from build123d import *

# Parameters (mm, degrees)
BOSS_EXTRUDE1_DEPTH = 0.254
SKETCH2_R           = 4.699
CUT_EXTRUDE1_DEPTH  = 1.254
SKETCH3_W           = 2.54
SKETCH3_H           = 0.635
CUT_EXTRUDE2_DEPTH  = 1.254
SKETCH5_OUTSIDE_W   = 121.447
SKETCH5_OUTSIDE_H   = 109.618
CUT_EXTRUDE5_DEPTH  = 1.254


with BuildPart() as part:
    # Sketch1 → Boss-Extrude1 (new body)
    with BuildSketch(Plane.XY):
        with BuildLine():
            Line((67.21146711, 76.191723231), (8.696654013, 17.676910134))
            Line((8.696654013, 17.676910134), (7.228954972, 14.133571205))
            ThreePointArc((7.228954972, 14.133571205), (14.666587579, 6.075099489), (15.105587123, -4.88230096))
            Line((15.105587123, -4.88230096), (18.648926052, -6.35))
            Line((18.648926052, -6.35), (101.401368334, -6.35))
            ThreePointArc((101.401368334, -6.35), (93.866160503, 38.880636728), (67.21146711, 76.191723231))
        make_face()
        with BuildLine():
            Line((88.672924278, 6.35), (27.86051193, 6.35))
            ThreePointArc((27.86051193, 6.35), (26.399857642, 10.93517908), (24.190484974, 15.210228852))
            Line((24.190484974, 15.210228852), (67.191354125, 58.211098004))
            ThreePointArc((67.191354125, 58.211098004), (82.13289044, 34.020557137), (88.672924278, 6.35))
        make_face(mode=Mode.SUBTRACT)
    extrude(amount=BOSS_EXTRUDE1_DEPTH)

    # Sketch2 → Cut-Extrude1 (cut, through all)
    with BuildSketch(Plane.XY.offset(0.254)):
        with Locations((22.225, 0)):
            Circle(SKETCH2_R)
        with Locations((36.195, 0)):
            Circle(SKETCH2_R)
        with Locations((61.722, 0)):
            Circle(SKETCH2_R)
        with Locations((75.692, 0)):
            Circle(SKETCH2_R)
        with Locations((95.25, 0)):
            Circle(SKETCH2_R)
        with Locations((15.715448212, 15.715448212)):
            Circle(SKETCH2_R)
        with Locations((25.593729945, 25.593729945)):
            Circle(SKETCH2_R)
        with Locations((43.644044748, 43.644044748)):
            Circle(SKETCH2_R)
        with Locations((53.522326482, 53.522326482)):
            Circle(SKETCH2_R)
        with Locations((92.004434954, 24.652514046)):
            Circle(SKETCH2_R)
        with Locations((82.48891971, 47.625)):
            Circle(SKETCH2_R)
        with Locations((67.351920908, 67.351920908)):
            Circle(SKETCH2_R)
    extrude(amount=-CUT_EXTRUDE1_DEPTH, mode=Mode.SUBTRACT)

    # Sketch3 → Cut-Extrude2 (cut, through all)
    with BuildSketch(Plane.XY.offset(0.254)):
        Polygon((15.266435406, 24.246691527), (17.06248663, 26.042742751), (17.511499436, 25.593729945), (15.715448212, 23.797678721), align=None)
        Polygon((44.991083167, 53.971339288), (43.195031942, 52.175288063), (43.644044748, 51.726275257), (45.440095973, 53.522326482), align=None)
        with Locations((29.21, -6.0325)):
            Rectangle(SKETCH3_W, SKETCH3_H)
        with Locations((68.707, -6.0325)):
            Rectangle(SKETCH3_W, SKETCH3_H)
        Polygon((29.230733674, 38.210989795), (31.026784898, 40.007041019), (31.475797704, 39.558028213), (29.67974648, 37.761976989), align=None)
        Polygon((56.845021246, 65.825277367), (55.048970022, 64.029226143), (55.497982828, 63.580213337), (57.294034052, 65.376264561), align=None)
        with Locations((48.9585, -6.0325)):
            Rectangle(SKETCH3_W, SKETCH3_H)
        with Locations((85.471, -6.0325)):
            Rectangle(SKETCH3_W, SKETCH3_H)
        Polygon((99.935462164, 14.437711971), (100.266998693, 11.919442024), (101.526133667, 12.085210288), (101.194597138, 14.603480236), align=None)
        Polygon((93.765504959, 37.464305742), (94.938831965, 37.950313702), (93.966816047, 40.296967714), (92.793489041, 39.810959755), align=None)
        Polygon((79.327792988, 62.471156422), (80.874047017, 60.456038938), (81.88160576, 61.229165953), (80.33535173, 63.244283437), align=None)
        Polygon((13.593916116, 7.005422516), (14.565932035, 4.658768503), (15.739259041, 5.144776462), (14.767243123, 7.491430475), align=None)
    extrude(amount=-CUT_EXTRUDE2_DEPTH, mode=Mode.SUBTRACT)

    # Sketch5 outside → Cut-Extrude5 (cut, through all)
    with BuildSketch(Plane.XY.offset(0.254)):
        with Locations((54.4145, 34.921)):
            Rectangle(SKETCH5_OUTSIDE_W, SKETCH5_OUTSIDE_H)
        Polygon((86.741, -7.62), (86.741, 10.138710513), (102.87, 12.262133647), (102.87, -7.62), align=None, mode=Mode.SUBTRACT)
    extrude(amount=-CUT_EXTRUDE5_DEPTH, mode=Mode.SUBTRACT)


solid = part.part
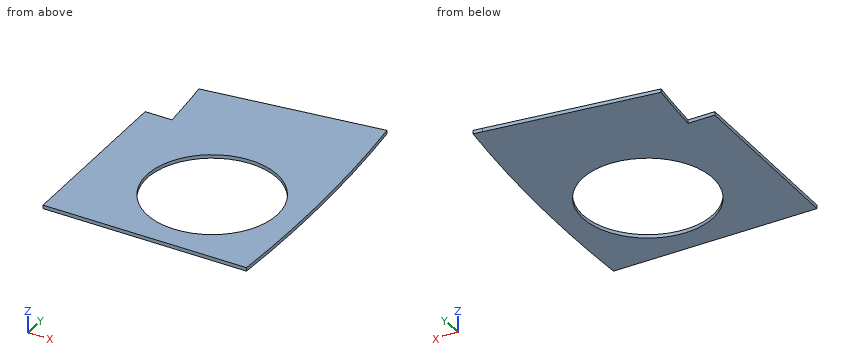
Design review of the part built by this model. Coordinates are the model's own, in mm. Round coordinates to 2 decimals unless told otherwise and drop trailing zeros. Order: outer loops, then holes, each group sorted by start corner. A loop starts at its lowest first (then second) coordinate and runs counter-clockwise, first axis right, second up.
1) Consider section B-B (z = 0.2). State the section outline as (x, y) points.
The answers:
outline: (86.74, -6.35) - (101.4, -6.35) arc R101.6 ccw to (100.89, 12) - (88.3, 10.34) arc R88.9 cw to (88.67, 6.35) - (86.74, 6.35) - close; hole circle Ø9.4 at (95.25, 0)
2) Consider section C-C (x = 95.25). State the section outline as (y, z) points.
The answers:
outline: (-6.35, 0) - (-4.7, 0) - (-4.7, 0.25) - (-6.35, 0.25) - close; (4.7, 0) - (11.26, 0) - (11.26, 0.25) - (4.7, 0.25) - close
3) For L1, parallel to Y at x = 96.25, z = 0.1; L2, parallel to X at y = 0.75, z = 0.2; L3, parallel to Y at x = 94, z = 0.2, list the stretches that pass through material, from the lowest coordinate up.
The answers:
L1: y = -6.35 to -4.59, 4.59 to 11.39
L2: x = 86.74 to 90.61, 99.89 to 101.6
L3: y = -6.35 to -4.53, 4.53 to 11.09
4) Clearance check with a flat-ended pin moving along its axis: pin 1 Ø6 at (x, y) = (95, 6) entering from -Z. State where the tip first meets the part, or that it passes through.
The answers:
pin 1: stops at z = 0
5) Consider section A-A (y = 0). State the section outline as (x, z) points, plus the area to 3 significant figures.
The answers:
outline: (86.74, 0) - (90.55, 0) - (90.55, 0.25) - (86.74, 0.25) - close; (99.95, 0) - (101.6, 0) - (101.6, 0.25) - (99.95, 0.25) - close
area: 1.39 mm2
